from build123d import *

# Parameters (mm, degrees)
SKETCH1_W           = 15
SKETCH1_H           = 30
BOSS_EXTRUDE1_DEPTH = 15
SKETCH2_W           = 25
SKETCH2_H           = 40
BOSS_EXTRUDE2_DEPTH = 1.5
SKETCH4_W           = 2
SKETCH4_H           = 2
CUT_EXTRUDE2_DEPTH  = 3
FILLET2_R           = 8


with BuildPart() as part:
    # Sketch1 → Boss-Extrude1 (new body)
    with BuildSketch(Plane(origin=(0, 0, 0), x_dir=(1, 0, 0), z_dir=(0, 1, 0))):
        with Locations((7.5, 15)):
            Rectangle(SKETCH1_W, SKETCH1_H)
        Polygon((2, 2), (13, 2), (13, 7.25), (13.25, 7.25), (13.25, 8.75), (13, 8.75), (13, 28), (2, 28), (2, 8.75), (1.75, 8.75), (1.75, 7.25), (2, 7.25), align=None, mode=Mode.SUBTRACT)
    extrude(amount=BOSS_EXTRUDE1_DEPTH)

    # Sketch2 → Boss-Extrude2 (add)
    with BuildSketch(Plane.XZ):
        with Locations((7.5, -15)):
            Rectangle(SKETCH2_W, SKETCH2_H)
    extrude(amount=BOSS_EXTRUDE2_DEPTH)

    # Sketch4 → Cut-Extrude2 (cut)
    with BuildSketch(Plane(origin=(0, 15, 0), x_dir=(1, 0, 0), z_dir=(0, 1, 0))):
        with Locations((8.5, 29)):
            Rectangle(SKETCH4_W, SKETCH4_H)
        with Locations((6.5, 1)):
            Rectangle(SKETCH4_W, SKETCH4_H)
    extrude(amount=-CUT_EXTRUDE2_DEPTH, mode=Mode.SUBTRACT)

    # Fillet2
    fillet2_edges = [part.edges().sort_by_distance(p)[0] for p in [
        (-5, -0.75, 5),
        (-5, -0.75, -35),
        (20, -0.75, -35),
        (20, -0.75, 5),
    ]]
    fillet(fillet2_edges, radius=FILLET2_R)


solid = part.part
The listing builds one solid part. Answer for the finished solid, in the listing's coordinates (mm). A direction names the side the tool comes from. Coordinates: 2 decimals unless noted, no trailing zeros. Loops run counter-clockwise (first coordinate to the right, second up) from the corner with the lowest first, then second, coordinate; pieces in that order, holes last.
1) Find section A-A on y = 9.5. Write down the section's boundary in (x, z), then the cut area to 3 significant figures.
2) Find section B-B on x = 6. Write down the section's boundary in (y, z).
3) Find section D-D on x = 14.25. Write down the section's boundary in (y, z).
4) Flat-ended cylindrical pins translate along their axes: pin 1 Ø9 at (x, y) = (6, 11) entering from -Z; pin 2 Ø1.2 at (y, z) = (6, -8) entering from -X; pin 3 Ø3.5 at (x, y) = (7.5, 11) entering from +Z. Find the tip coordinate at first contact, or state that the pin passes through.
5) A tool of negligible diameter and unlimited length cuts with its end or side. For faces 4 (the face through (13.25, 7, -8)), 5 (the face through (15, 7, -15)), 6 (the face through (9.5, 14, -29)), from which of +Z, -Z, +X, -X, +Y, -Y can it reach the whole face along a straight path? Write none if from no direction.
6) Determine the mould class of faces 1 (the face through (8, 7, -28)), 2 (the face through (0, 7, -15)), 3 (the face through (7, 7, -30)) for opening direction Z: pulls with the +Z half, pulls with the -Z half, needs draft (parallel to the pull), parting line crosses it, or undercut.
7) Find section C-C on z = -9.5. Write down the section's boundary in (x, y), then the cut area to 3 significant figures.
8) Find the intervals of material crossed by L1, parallel to Z at x = 11, y = 6; L2, parallel to X at y = 4.75, z = -13; L3, parallel to Y at x = -3, z = -32, in increasing order.
Values:
1. outline: (0, -30) - (15, -30) - (15, 0) - (0, 0) - close; hole (1.75, -8.75) - (2, -8.75) - (2, -28) - (13, -28) - (13, -8.75) - (13.25, -8.75) - (13.25, -7.25) - (13, -7.25) - (13, -2) - (2, -2) - (2, -7.25) - (1.75, -7.25) - close
1. area: 163 mm2
2. outline: (-1.5, -35) - (0, -35) - (0, -30) - (15, -30) - (15, -28) - (0, -28) - (0, -2) - (12, -2) - (12, 0) - (0, 0) - (0, 5) - (-1.5, 5) - close
3. outline: (-1.5, -34.68) - (0, -34.68) - (0, -30) - (15, -30) - (15, 0) - (0, 0) - (0, 4.68) - (-1.5, 4.68) - close
4. pin 1: stops at z = -30
4. pin 2: stops at x = 0
4. pin 3: stops at z = 0
5. face 4: +Y
5. face 5: +Z, -Z, +X, +Y
5. face 6: -Z, +Y
6. face 1: undercut
6. face 2: needs draft
6. face 3: pulls with the -Z half
7. outline: (-5, -1.5) - (20, -1.5) - (20, 0) - (15, 0) - (15, 15) - (13, 15) - (13, 0) - (2, 0) - (2, 15) - (0, 15) - (0, 0) - (-5, 0) - close
7. area: 97.5 mm2
8. L1: z = -30 to -28, -2 to 0
8. L2: x = 0 to 2, 13 to 15
8. L3: y = -1.5 to 0
